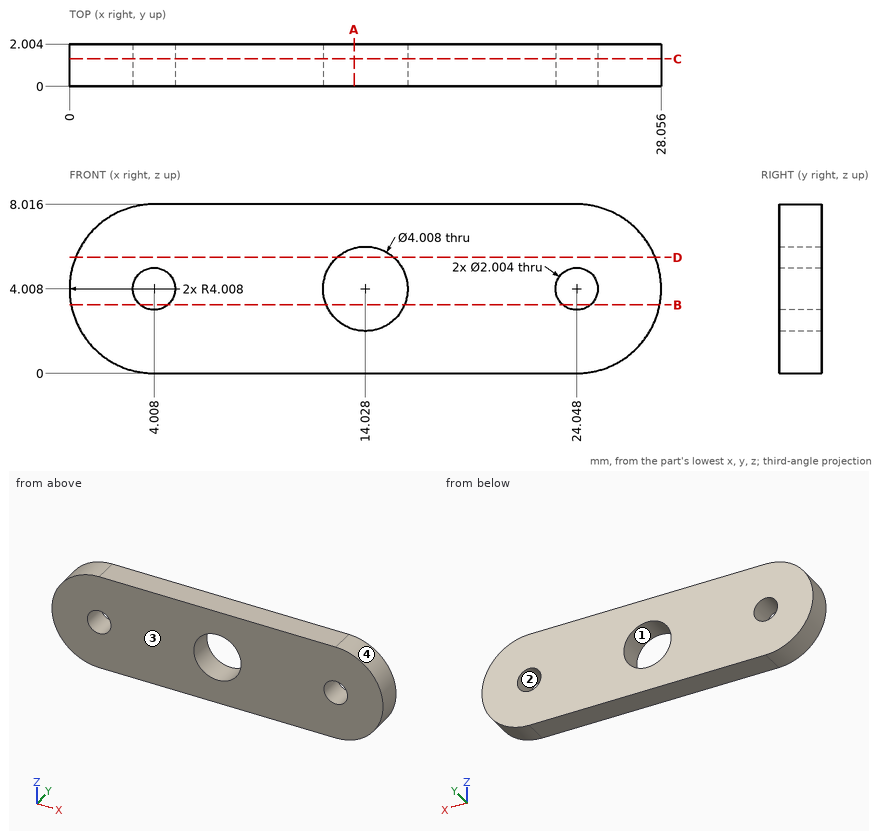
Source: three-view drawing plus pictorial views. Frame: mm from the lowest corner of the part. Round coordinates to 2 decimals unless told otherwise and drop trailing zeros. Write each loop counter-clockwise with the first axis right and the second up, starting at its lowest first coordinate (ties: lowest second). Pieces come first, ordered by that corner, then holes. Notation, with made-up numbers: M 85.25,24 L 110.25,24 A8 ccw 110.25,39 Z; hole C 18.25,-2 d5. An arc over 180 degrees is marked long. Write item = value, one per line.
Item 1: Material intervals for line 1 along Z through (x, y) = (14, 1.1); line 2 along X through (y, z) = (1.4, 3.25); line 3 along X through (y, z) = (1.1, 4.25), sorted ascending. Write a range as [from, to].
Findings:
line_1 = [0, 2], [6.01, 8.02]
line_2 = [0.07, 3.35], [4.66, 12.17], [15.88, 23.39], [24.7, 27.98]
line_3 = [0.01, 3.04], [4.98, 12.04], [16.02, 23.08], [25.02, 28.05]
Item 2: Section query B-B on z = 3.25. Return loops of the section in (x, y), then the cut area to 3 significant figures.
Findings:
outline = M 0.07,0 L 3.35,0 L 3.35,2 L 0.07,2 Z; M 4.66,0 L 12.17,0 L 12.17,2 L 4.66,2 Z; M 15.88,0 L 23.39,0 L 23.39,2 L 15.88,2 Z; M 24.7,0 L 27.98,0 L 27.98,2 L 24.7,2 Z
area = 43.2 mm^2
Item 3: Section query A-A on x = 13.5. Return loops of the section in (y, z), then the cut area to 3 significant figures.
Findings:
outline = M 0,0 L 2,0 L 2,2.07 L 0,2.07 Z; M 0,5.94 L 2,5.94 L 2,8.02 L 0,8.02 Z
area = 8.32 mm^2
Item 4: Pin query (flat end, axial travel): P1, Ø1.6, axis at x = 4.008, z = 4.008, coming from the -Y side. Return the tip coordinate at first contact, or that it passes through.
Findings:
P1 = through
Item 5: Pull-direction query (X, two-part tool) for the marked faces 1, 2, 3 and 4; classes: pulls with the +X half, pulls with the -X half, needs draft (parallel to the pull), parting line crosses it, or undercut.
Findings:
face_1 = undercut
face_2 = undercut
face_3 = needs draft
face_4 = pulls with the +X half
Item 6: Section query D-D on z = 5.5. Return loops of the section in (x, y), then the cut area to 3 significant figures.
Findings:
outline = M 0.29,0 L 12.69,0 L 12.69,2 L 0.29,2 Z; M 15.37,0 L 27.77,0 L 27.77,2 L 15.37,2 Z
area = 49.7 mm^2
Item 7: Section query C-C on y = 1.3. Return loops of the section in (x, z), then the cut area to 3 significant figures.
Findings:
outline = M 4.01,0 L 24.05,0 A4.01 ccw 24.05,8.02 L 4.01,8.02 A4.01 ccw Z; hole C 4.01,4.01 d2; hole C 14.03,4.01 d4.01; hole C 24.05,4.01 d2
area = 192 mm^2
